```python
from build123d import *

# Parameters (mm, degrees)
BOSS_EXTRUDE2_DEPTH = 20
SKETCH2_W           = 15
SKETCH2_H           = 100
BOSS_EXTRUDE3_DEPTH = 12


with BuildPart() as part:
    # Sketch1 → Boss-Extrude2 (new body)
    with BuildSketch(Plane.XY):
        Polygon((87.329047187, 46.385009916), (-62.670952813, 46.385009916), (-62.670952813, -118.614990084), (-50.670952813, -118.614990084), (-50.670952813, -3.614990084), (-15.670952813, 31.385009916), (40.329047187, 31.385009916), (75.329047187, -3.614990084), (75.329047187, -8.614990084), (87.329047187, -8.614990084), align=None)
        Polygon((75.329047187, 11.385009916), (55.329047187, 31.385009916), (75.329047187, 31.385009916), align=None, mode=Mode.SUBTRACT)
        Polygon((-50.670952813, 31.385009916), (-30.670952813, 31.385009916), (-50.670952813, 11.385009916), align=None, mode=Mode.SUBTRACT)
    extrude(amount=BOSS_EXTRUDE2_DEPTH)

    # Sketch2 → Boss-Extrude3 (add)
    with BuildSketch(Plane(origin=(87.329047187, 0, 0), x_dir=(0, 0, -1), z_dir=(1, 0, 0))):
        Polygon((-20, -8.614990084), (-63.858795675, -8.614990084), (-63.858795675, -41.914961686), (51.271272263, -41.914961686), (51.271272263, -8.614990084), (0, -8.614990084), align=None)
        Polygon((-63.858795675, -41.914961686), (-63.858795675, -8.614990084), (-78.858795675, -8.614990084), (-78.858795675, -108.614990084), (-63.858795675, -108.614990084), align=None)
        with Locations((58.771272263, -58.614990084)):
            Rectangle(SKETCH2_W, SKETCH2_H)
    extrude(amount=-BOSS_EXTRUDE3_DEPTH)


solid = part.part
```
Build history of the part. All positions in model axes, mm. A direction names the side the tool comes from. Give positions to 0.01 mm unless a question says otherwise; leave off trailing zeros. Loops run counter-clockwise (first coordinate to the right, second up) from the corner with the lowest first, then second, coordinate; pieces in that order, holes last.
1) Probe line 1 along Y through (x, z) = (20.5, 6.5) (3 decimals); line 2 along X through (y, z) = (-23.5, 37.5); line 3 along Z through (x, y) = (49.5, 33). List the from-to ranges inside material, lowest first.
Values follow:
line 1: y = 31.385 to 46.385
line 2: x = 75.33 to 87.33
line 3: z = 0 to 20
2) Band-saw the part on D-D on y = 22. List the corners of the cut face in (x, z).
Values follow:
outline: (-62.67, 0) - (-50.67, 0) - (-50.67, 20) - (-62.67, 20) - close; (-40.06, 0) - (-25.06, 0) - (-25.06, 20) - (-40.06, 20) - close; (49.71, 0) - (64.71, 0) - (64.71, 20) - (49.71, 20) - close; (75.33, 0) - (87.33, 0) - (87.33, 20) - (75.33, 20) - close
3) Two-plate mould, pull along Y, no slides. Class faces 5 (the face through (81, -41.915, 7)), 6 (the face through (-50.671, 21, 10)), 7 (the face through (-21, 31, 20)), 8 (the face through (65.469, 21.245, 9.86)): released by +Y, released by -Y, zero draft, split by the parting line, or undercut.
Values follow:
face 5: released by -Y
face 6: undercut
face 7: zero draft
face 8: undercut
4) 3-axis set-ups, long thin cutter, end or side, ignore diameter. For faces 1 (the face through (-50.671, -62, 10)), 2 (the face through (65, 31.385, 10)), 3 (the face through (81, -58, 78.859)), 4 (the face through (81, -76, -51.271)): which of +Z, -Z, +X, -X, +Y, -Y reach the whole face in a straight line?
Values follow:
face 1: +Z, -Z, -Y
face 2: +Z, -Z
face 3: +Z, +X, -X, +Y, -Y
face 4: +X, -X, -Y
5) Drop flat-ended pins along their axis: P1, Ø4, axis at y = -35.5, z = 41, coming from the -X side; P2, Ø3.5, axis at x = 78.5, z = -58, coming from the -Y side (3 decimals); P3, Ø9.5, axis at x = 79, z = -4, coming from the -Y side; P4, Ø22, axis at x = -44, z = 12, coming from the -Y side (3 decimals). Give the stop position or say it passes through.
Values follow:
P1: stops at x = 75.33
P2: stops at y = -108.615
P3: stops at y = -41.91
P4: stops at y = -118.615
6) Band-saw the part on C-C on y = -22. List the corners of the cut face in (x, z).
Values follow:
outline: (-62.67, 0) - (-50.67, 0) - (-50.67, 20) - (-62.67, 20) - close; (75.33, -66.27) - (87.33, -66.27) - (87.33, 78.86) - (75.33, 78.86) - close
7) Band-saw the part on A-A on y = -75.5. List the corners of the cut face in (x, z), then the cut area to 3 significant figures.
Values follow:
outline: (-62.67, 0) - (-50.67, 0) - (-50.67, 20) - (-62.67, 20) - close; (75.33, -66.27) - (87.33, -66.27) - (87.33, -51.27) - (75.33, -51.27) - close; (75.33, 63.86) - (87.33, 63.86) - (87.33, 78.86) - (75.33, 78.86) - close
area: 600 mm2
8) Band-saw the part on B-B on z = 13. List the corners of the cut face in (x, y) (3 decimals), then the cut area to 3 significant figures.
Values follow:
outline: (-62.671, -118.615) - (-50.671, -118.615) - (-50.671, -3.615) - (-15.671, 31.385) - (40.329, 31.385) - (75.329, -3.615) - (75.329, -41.915) - (87.329, -41.915) - (87.329, 46.385) - (-62.671, 46.385) - close; hole (-50.671, 11.385) - (-30.671, 31.385) - (-50.671, 31.385) - close; hole (55.329, 31.385) - (75.329, 11.385) - (75.329, 31.385) - close
area: 5,750 mm2
